Geometry check sheet. Reference: the model listing, model coordinates, mm. Face numbers are marked on the shaded views. A direction names the side the tool comes from. Round coordinates to 2 decimals unless told otherwise and drop trailing zeros. Write each loop counter-clockwise with the first axis right and the second up, starting at its lowest first coordinate (ties: lowest second). Pieces come first, ordered by that corner, then holes.
Item 1: Cross-section at C-C (z = 6.25). Enter the section's corners in (x, y), then the cut area to 3 significant figures.
Item 2: Draft check along X on the marked faces 1, 2, 3 and 4. Enter one of: pulls with the +X half, pulls with the -X half, needs draft (parallel to the pull), parting line crosses it, or undercut.
Item 3: Scan lines: probe 1 along Y at (x, z) = (0, 5.2); probe 2 along Y at (x, z) = (0, 0.2); probe 3 along Y at (x, z) = (0, 0.35). Record each from-to range of solid material in increasing order.
Item 4: Depth check by flat-ended pin: P1, Ø12, axis at x = 2.5, y = 7.5, coming from the -Z side; P2, Ø3.5, axis at x = 0, y = 0, coming from the -Z side; P3, Ø1, axis at x = 4.5, z = 1, coming from the -Y side; P4, Ø1.5, axis at y = 4, z = 6, coming from the -X side. Enter the tip coordinate at first touch or a pass-through.
Item 5: Access from +Z, -Z, +X, -X, +Y, -Y to the whole of each face (thin tool, end or side, straight path). Record for the marked faces 5, 6 and 7.
from build123d import *

# Parameters (mm, degrees)
F0_R     = 4
F0_R_2   = 2
F1_DEPTH = 7
F0_R_3   = 6
F2_DEPTH = 4
F0_R_4   = 11
F3_DEPTH = 3
F4_DEPTH = 4
F5_R     = 2
F6_DEPTH = 0.5


with BuildPart() as f1:
    # F0 (on Top) → F1 (new body)
    with BuildSketch(Plane.XY):
        Circle(F0_R)
        Circle(F0_R_2, mode=Mode.SUBTRACT)
    extrude(amount=F1_DEPTH)

    # F0 (on Top) → F2 (join)
    with BuildSketch(Plane.XY):
        Circle(F0_R_3)
        Circle(F0_R, mode=Mode.SUBTRACT)
    extrude(amount=F2_DEPTH)

    # F0 (on Top) → F3 (join)
    with BuildSketch(Plane.XY):
        Circle(F0_R_4)
        Circle(F0_R_3, mode=Mode.SUBTRACT)
    extrude(amount=F3_DEPTH)

    # F0 (on Top) → F4 (join)
    with BuildSketch(Plane.XY):
        Circle(F0_R_2)
    extrude(amount=F4_DEPTH)

    # F5
    f5_edges = [f1.edges().sort_by_distance(p)[0] for p in [
        (-11, 0, 0),
    ]]
    fillet(f5_edges, radius=F5_R)

    # F0 (on Top) → F6 (cut)
    with BuildSketch(Plane.XY):
        Circle(F0_R_3)
        Circle(F0_R, mode=Mode.SUBTRACT)
        Circle(F0_R_2)
    extrude(amount=F6_DEPTH, mode=Mode.SUBTRACT)


solid = f1.part
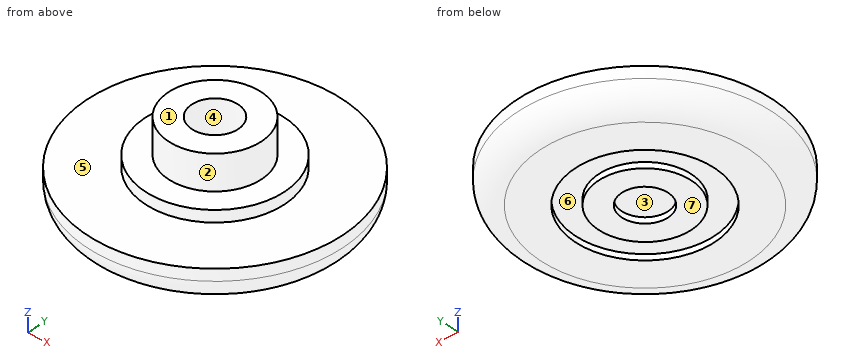
Resolved:
1. outline: circle Ø8 at (0, 0); hole circle Ø4 at (0, 0)
1. area: 37.7 mm2
2. face 1: needs draft
2. face 2: parting line crosses it
2. face 3: undercut
2. face 4: undercut
3. probe 1: y = -4 to -2, 2 to 4
3. probe 2: y = -9.87 to -6, -4 to -2, 2 to 4, 6 to 9.87
3. probe 3: y = -10.13 to -6, -4 to -2, 2 to 4, 6 to 10.13
4. P1: stops at z = 0
4. P2: stops at z = 0.5
4. P3: stops at y = -10.07
4. P4: stops at x = -2.33
5. face 5: +Z
5. face 6: -Z
5. face 7: -Z, +X, -X, +Y, -Y
